Autodesk Inventor part; units mm, degrees
ref_plane "YZ Plane" through (0, 0, 0) normal (1, 0, 0) x (0, 1, 0)
ref_plane "XZ Plane" through (0, 0, 0) normal (0, 1, 0) x (-1, 0, 0)
ref_plane "XY Plane" through (0, 0, 0) normal (0, 0, 1) x (1, 0, 0)
sketch "Sketch1" plane through (0, 0, 0) normal (0, 0, 1) x (1, 0, 0)
  line L0 (-35.2109, 0) -> (35.2109, 0) construction
  line L1 (0, -35.2109) -> (0, 35.2109) construction
  line L2 (0, 0) -> (13.4339, 13.4339) construction
  line L3 (0, 0) -> (18.9985, 0) construction
  line L4 (0, 25.1006) -> (17, 25.1006)
  line L5 (17, 25.1006) -> (17, 21.4406)
  line L6 (17, 21.4406) -> (19.2203, 19.2203)
  line L7 (25.1006, 0) -> (25.1006, 17)
  line L8 (25.1006, 17) -> (21.4406, 17)
  line L9 (21.4406, 17) -> (19.2203, 19.2203)
  line L10 (0, 0) -> (-13.4339, 13.4339) construction
  line L11 (0, 0) -> (-18.9985, 0) construction
  line L12 (0, 25.1006) -> (-17, 25.1006)
  line L13 (-17, 25.1006) -> (-17, 21.4406)
  line L14 (-17, 21.4406) -> (-19.2203, 19.2203)
  line L15 (-25.1006, 0) -> (-25.1006, 17)
  line L16 (-25.1006, 17) -> (-21.4406, 17)
  line L17 (-21.4406, 17) -> (-19.2203, 19.2203)
  line L18 (0, 0) -> (13.4339, -13.4339) construction
  line L19 (0, -25.1006) -> (17, -25.1006)
  line L20 (17, -25.1006) -> (17, -21.4406)
  line L21 (17, -21.4406) -> (19.2203, -19.2203)
  line L22 (25.1006, 0) -> (25.1006, -17)
  line L23 (25.1006, -17) -> (21.4406, -17)
  line L24 (21.4406, -17) -> (19.2203, -19.2203)
  line L25 (0, 0) -> (-13.4339, -13.4339) construction
  line L26 (0, -25.1006) -> (-17, -25.1006)
  line L27 (-17, -25.1006) -> (-17, -21.4406)
  line L28 (-17, -21.4406) -> (-19.2203, -19.2203)
  line L29 (-25.1006, 0) -> (-25.1006, -17)
  line L30 (-25.1006, -17) -> (-21.4406, -17)
  line L31 (-21.4406, -17) -> (-19.2203, -19.2203)
  line L32 (-17.05, 25.1506) -> (0, 25.1506)
  line L33 (0, 25.1506) -> (17.05, 25.1506)
  line L34 (17.05, 25.1506) -> (17.05, 21.4613)
  line L35 (17.05, 21.4613) -> (19.2557, 19.2557)
  line L36 (19.2557, 19.2557) -> (21.4613, 17.05)
  line L37 (21.4613, 17.05) -> (25.1506, 17.05)
  line L38 (25.1506, 17.05) -> (25.1506, 0)
  line L39 (25.1506, 0) -> (25.1506, -17.05)
  line L40 (25.1506, -17.05) -> (21.4613, -17.05)
  line L41 (21.4613, -17.05) -> (19.2557, -19.2557)
  line L42 (19.2557, -19.2557) -> (17.05, -21.4613)
  line L43 (17.05, -21.4613) -> (17.05, -25.1506)
  line L44 (17.05, -25.1506) -> (0, -25.1506)
  line L45 (0, -25.1506) -> (-17.05, -25.1506)
  line L46 (-17.05, -25.1506) -> (-17.05, -21.4613)
  line L47 (-17.05, -21.4613) -> (-19.2557, -19.2557)
  line L48 (-19.2557, -19.2557) -> (-21.4613, -17.05)
  line L49 (-21.4613, -17.05) -> (-25.1506, -17.05)
  line L50 (-25.1506, -17.05) -> (-25.1506, 0)
  line L51 (-25.1506, 0) -> (-25.1506, 17.05)
  line L52 (-25.1506, 17.05) -> (-21.4613, 17.05)
  line L53 (-21.4613, 17.05) -> (-19.2557, 19.2557)
  line L54 (-19.2557, 19.2557) -> (-17.05, 21.4613)
  line L55 (-17.05, 21.4613) -> (-17.05, 25.1506)
  dimension "d0" = 45
  dimension "d1" = 3.14
  dimension "d2" = 3.66
  dimension "d3" = 17
  dimension "d23" = 0.05
extrude "Extrusion1" add sketch "Sketch1" along normal blind 8 contours L4 L5 L6 L9 L8 L7 L22 L23 L24 L21 L20 L19 L26 L27 L28 L31 L30 L29 L15 L16 L17 L14 L13 L12 | L32 L33 L34 L35 L36 L37 L38 L39 L40 L41 L42 L43 L44 L45 L46 L47 L48 L49 L50 L51 L52 L53 L54 L55
hole "Hole1" at (0, 0, 0) direction (0, 0, 1) diameter 30 end through all
sketch "Sketch2" plane through (0, 0, 0) normal (0, 0, -1) x (-1, 0, 0)
  circle A0 centre (0, 0) radius 15
  line L0 (3.1688, 14.6615) -> (14.2816, -4.5865)
  line L1 (11.1128, -10.075) -> (-11.1128, -10.075)
  line L2 (-14.2816, -4.5865) -> (-3.1688, 14.6615)
  circle A1 centre (0, 0) radius 10.075 construction
  circle A2 centre (0, 0) radius 15 construction
  circle A3 centre (0, 0) radius 15 construction
  arc A4 (14.2816, -4.5865) -> (3.1688, 14.6615) centre (0, 0) ccw
  arc A5 (-11.1128, -10.075) -> (11.1128, -10.075) centre (0, 0) ccw
  arc A6 (-3.1688, 14.6615) -> (-14.2816, -4.5865) centre (0, 0) ccw
  dimension "d22" = 20.15
extrude "Extrusion2" add sketch "Sketch2" against normal up to surface (8 mm away) contours A0 L0 | L2 A0 | A0 L1
equation "\"Lens_diameter\" = 25"
properties part number "20_IM_Cube_Insert_Lens_holder_RMS_63x"
Geometry check sheet. Reference: the model listing, model coordinates, mm. A direction names the side the tool comes from. Round coordinates to 2 decimals unless told otherwise and drop trailing zeros. Order: outer loops, then holes, each group sorted by start corner. A loop starts at its lowest first (then second) coordinate and runs counter-clockwise, first axis right, second up. Notation, with made-up numbers: (-36, -29.5) -> (20, -29.5) arc R14 ccw to (20, -14.5) -> close; hole circle Ø8 at (9.5, 0). An arc over 180 degrees is marked (long way). Use one line per item in the form item = value.
1. Mould release check, pull along Y, two halves, no side actions. Record for faces 4 (the face through (-25.151, 0, 4)), 5 (the face through (-23, 17.05, 4)), 6 (the face through (-13.013, -7.461, 4.056)), 7 (the face through (0, 15, 4)): pulls with the +Y half, pulls with the -Y half, needs draft (parallel to the pull), parting line crosses it, or undercut.
Working result:
face_4 = needs draft
face_5 = pulls with the +Y half
face_6 = undercut
face_7 = undercut
2. Cross-section at C-C, the plane y = 1. Enter the section's corners in (x, z).
Working result:
outline = (-25.15, 0) -> (-11.06, 0) -> (-11.06, 8) -> (-25.15, 8) -> close; (11.06, 0) -> (25.15, 0) -> (25.15, 8) -> (11.06, 8) -> close
3. Cross-section at D-D, the plane y = 18. Enter the section's corners in (x, z), plus the area to 3 significant figures.
Working result:
outline = (-20.51, 0) -> (20.51, 0) -> (20.51, 8) -> (-20.51, 8) -> close
area = 328 mm^2
4. Set-up check for faces 1 (the face through (-8.65, 5.17, 3.94)), 2 (the face through (-17.05, -23, 4)), 3 (the face through (23, -17.05, 4)): record each of +Z, -Z, +X, -X, +Y, -Y from which the full face is reachable in a straight line by a thin tool's end or side.
Working result:
face_1 = +Z, -Z
face_2 = +Z, -Z, -X, -Y
face_3 = +Z, -Z, +X, -Y
5. Go/stop test with flat-tipped pins: pin 1 (1.8 mm diameter, centred on x = 23, z = 3.5, fed in from -Y); pin 2 (4 mm diameter, centred on y = 22.5, z = 4.5, fed in from +X); pin 3 (3 mm diameter, centred on y = 23, z = 4.5, fed in from -X). Record where each tip stops, or that it passes through.
Working result:
pin_1 = -17.05
pin_2 = 18.01
pin_3 = -17.05
6. Scan lines: line 1 along Y through (x, z) = (0, 2.75) (3 decimals); line 2 along Y through (x, z) = (-2, 5.5) (3 decimals); line 3 along X through (y, z) = (-9, 3.75). Record each from-to range of solid material in increasing order. Write a range as from..to.
Working result:
line_1 = -25.151..-10.075, 15..25.151
line_2 = -25.151..-10.075, 14.866..25.151
line_3 = -25.15..-12, 12..25.15
7. Cross-section at A-A, the plane x = 0. Enter the section's corners in (y, z) (3 decimals), plus the area to 3 significant figures.
Working result:
outline = (-25.151, 0) -> (-10.075, 0) -> (-10.075, 8) -> (-25.151, 8) -> close; (15, 0) -> (25.151, 0) -> (25.151, 8) -> (15, 8) -> close
area = 202 mm^2
